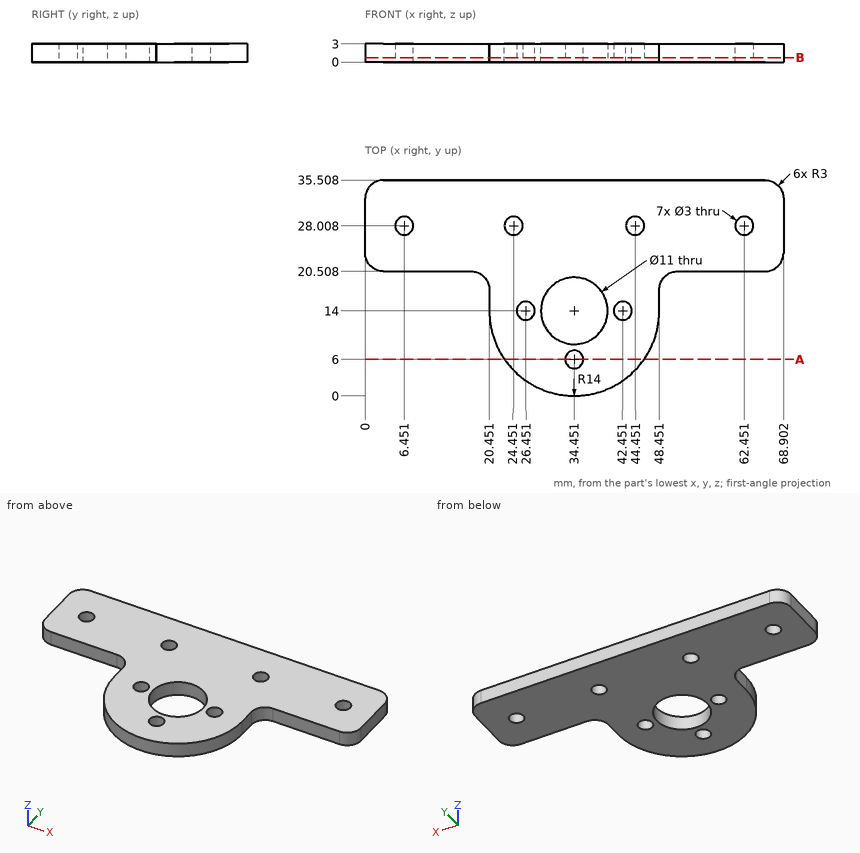
Study the drawing (mm; zero at the part's minimum x, y, z) and answer. Give positions to 0.01 mm unless a question says otherwise; leave off trailing zeros. Loops run counter-clockwise (first coordinate to the right, second up) from the corner with the lowest first, then second, coordinate; pieces in that order, holes last. Notation, with made-up numbers: (21, -12) - (67, -12) arc R34 ccw to (67, 22) - close; hole circle Ø1 at (48.25, -27.75). An arc over 180 degrees is marked (long way). Return JSON: item names as keys, results as strings. Group by question number.
1. Find section A-A (y = 6). Write down the section's boundary in (x, z).
2. Find section B-B (z = 0.75). State how many separate pieces and enclosed holes the cut face has.
3. Given pin 1 Ø2 at (x, y) = (47.5, 31) entering from -Z; pin 2 Ø1.5 at (y, z) = (16, 1.5) entering from -X; pin 3 Ø1.8 at (x, y) = (44.45, 28.01) entering from +Z, each flat-ended and moving along its own axis, determine where each tip first touches the part or whether it passes through.
4. Straight lines are drawn through the part: line 1 (X direction, y = 27, z = 2.35); line 2 (Y direction, x = 6.5, z = 1.65); line 3 (Y direction, x = 4.5, z = 2.45). For each, find the intervals that lie inside material, in ascending order. Write a range as [from, to].
Verdict:
{
 "1": {"outline": "(22.96, 0) - (32.95, 0) - (32.95, 3) - (22.96, 3) - close; (35.95, 0) - (45.94, 0) - (45.94, 3) - (35.95, 3) - close"},
 "2": {"separate pieces": "1", "enclosed holes": "8"},
 "3": {"pin 1": "stops at z = 0", "pin 2": "stops at x = 20.45", "pin 3": "passes through"},
 "4": {"line 1": "x = [0, 5.34], [7.56, 23.34], [25.56, 43.34], [45.56, 61.34], [63.56, 68.9]", "line 2": "y = [20.51, 26.51], [29.51, 35.51]", "line 3": "y = [20.51, 35.51]"}
}
